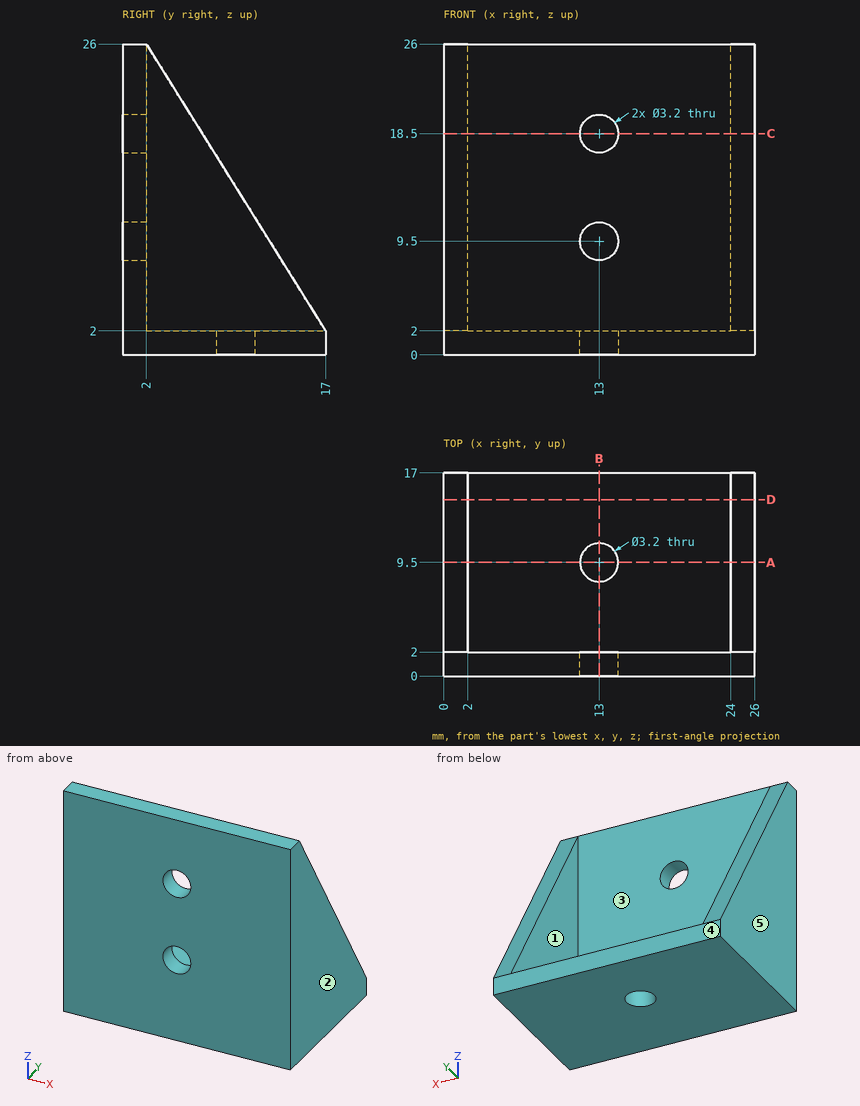
Verification items for this drawing (mm, ordinates from the low corner). A direction names the side the tool comes from. Give positions to 0.01 mm unless a question says otherwise; leave off trailing zeros. Write each loop counter-clockwise with the first axis right and the second up, starting at its lowest first coordinate (ties: lowest second). Pieces come first, ordered by that corner, then holes. Notation, with made-up numbers: (-7, 26) - (17, 26) arc R22 cw to (17, 37) - close; hole circle Ø11 at (-7.5, 58). An arc over 180 degrees is marked (long way). Answer as a JSON object with one key per item and string values. Group by question number.
1) Sectioned sample at A-A (y = 9.5). Record the cut outline in (x, z), then the cut area to 3 significant figures.
2) Thickness scan on probe 1 along X at (y, z) = (8, 12); probe 2 along Y at (x, z) = (13, 1.4); probe 3 along X at (y, z) = (0.7, 18.5). Record the ranges inside material, lowest first. Write a range as from..to.
3) Sectioned sample at B-B (x = 13). Record the cut outline in (y, z), then the cut area to 3 significant figures.
4) Access from +Z, -Z, +X, -X, +Y, -Y to the whole of each face (thin tool, end or side, straight path). Record for the marked faces 1 and 2.
5) Release check for a two-part mould opening along X. For the marked faces 3, 4 and 5 record: pulls with the +X half, pulls with the -X half, needs draft (parallel to the pull), parting line crosses it, or undercut.
6) Sectioned sample at D-D (y = 14.75). Record the cut outline in (x, z).
7) Depth check by flat-ended pin: P1, Ø4, axis at x = 19.5, z = 3, coming from the -Y side; P2, Ø7.5, axis at x = 9, y = 11.5, coming from the +Z side; P3, Ø4, axis at x = 13, z = 9.5, coming from the +Y side. Enter the tip coordinate at first touch or a pass-through.
8) Sectioned sample at C-C (z = 18.5). Record the cut outline in (x, y), then the cut area to 4 significant figures.
Geometry results:
{
 "1": {"outline": "(0, 0) - (11.4, 0) - (11.4, 2) - (2, 2) - (2, 14) - (0, 14) - close; (14.6, 0) - (26, 0) - (26, 14) - (24, 14) - (24, 2) - (14.6, 2) - close", "area": "93.6 mm^2"},
 "2": {"probe 1": "x = 0..2, 24..26", "probe 2": "y = 0..7.9, 11.1..17", "probe 3": "x = 0..11.4, 14.6..26"},
 "3": {"outline": "(0, 0) - (7.9, 0) - (7.9, 2) - (2, 2) - (2, 7.9) - (0, 7.9) - close; (0, 11.1) - (2, 11.1) - (2, 16.9) - (0, 16.9) - close; (0, 20.1) - (2, 20.1) - (2, 26) - (0, 26) - close; (11.1, 0) - (17, 0) - (17, 2) - (11.1, 2) - close", "area": "62.8 mm^2"},
 "4": {"face 1": "+Z, +Y", "face 2": "+Z, -Z, +X, +Y, -Y"},
 "5": {"face 3": "undercut", "face 4": "needs draft", "face 5": "pulls with the -X half"},
 "6": {"outline": "(0, 0) - (26, 0) - (26, 5.6) - (24, 5.6) - (24, 2) - (2, 2) - (2, 5.6) - (0, 5.6) - close"},
 "7": {"P1": "stops at y = 0", "P2": "stops at z = 2", "P3": "stops at y = 2"},
 "8": {"outline": "(0, 0) - (11.4, 0) - (11.4, 2) - (2, 2) - (2, 6.69) - (0, 6.69) - close; (14.6, 0) - (26, 0) - (26, 6.69) - (24, 6.69) - (24, 2) - (14.6, 2) - close", "area": "64.35 mm^2"}
}
